from build123d import *

# Parameters (mm, degrees)
SKETCH1_W           = 38.1
SKETCH1_H           = 17.78
SKETCH1_R           = 1.778
BOSS_EXTRUDE2_DEPTH = 3.175
BOSS_EXTRUDE3_DEPTH = 38.1


with BuildPart() as part:
    # Sketch1 → Boss-Extrude2 (new body)
    with BuildSketch(Plane.XY):
        with Locations((19.05, -8.89)):
            Rectangle(SKETCH1_W, SKETCH1_H)
        with Locations((5.579618, -11.929615714)):
            Circle(SKETCH1_R, mode=Mode.SUBTRACT)
        with Locations((32.520382, -11.929615714)):
            Circle(SKETCH1_R, mode=Mode.SUBTRACT)
    extrude(amount=BOSS_EXTRUDE2_DEPTH)

    # Sketch4 → Boss-Extrude3 (add)
    with BuildSketch(Plane(origin=(38.1, 0, 0), x_dir=(0, 0, -1), z_dir=(1, 0, 0))):
        Polygon((-3.175, -6.35), (-15.875, 0), (-3.175, 0), align=None)
    extrude(amount=-BOSS_EXTRUDE3_DEPTH)


solid = part.part
Build history of the part. All positions in model axes, mm. Round coordinates to 2 decimals unless told otherwise and drop trailing zeros. Write each loop counter-clockwise with the first axis right and the second up, starting at its lowest first coordinate (ties: lowest second). Pieces come first, ordered by that corner, then holes. Notation, with made-up numbers: M 14.5,40.25 L 68.5,40.25 A34 ccw 68.5,77.25 Z; hole C 2,67 d8. An arc over 180 degrees is marked long. Answer as a JSON object with one key per item and string values. Group by question number.
(1) Cut at D-D (z = 10.75). Give the cut face in (x, y), and give its area (3 significant figures).
(2) Cut at C-C (y = -16.25). Give the cut face in (x, z) (3 decimals).
(3) Mould opens along X. For faces 1 (the flat face through (19, -12, 3.175)), 2 (the flat face through (38.1, -5, 4)), 3 (the cylindrical face through (4.27, -10.73, 1.57)) say: pulls with the +X half, pulls with the -X half, needs draft (parallel to the pull), parting line crosses it, or undercut.
(4) Drill centre lines: L1, parallel to X at y = -11, z = 1.5; L2, parallel to Z at x = 20, y = -16.75 (3 decimals); L3, parallel to Y at x = 4, z = 1.5. Where is each one in solid material? Low to high.
(5) Cut at A-A (z = 2.75). Give the cut face in (x, y).
(6) Cut at B-B (x = 21). Give the cut face in (y, z) (3 decimals).
(7) Flat gauge pins, fed straight in: pin 1 (2 mm diameter, centred on x = 15, z = 4.5, fed in from -Y); pin 2 (2 mm diameter, centred on x = 32.52, y = -11.93, fed in from +Z). Where does each tip first touch, or does it go through?
Responses:
{
 "1": {"outline": "M 0,-2.56 L 38.1,-2.56 L 38.1,0 L 0,0 Z", "area": "97.6 mm2"},
 "2": {"outline": "M 0,0 L 38.1,0 L 38.1,3.175 L 0,3.175 Z"},
 "3": {"face 1": "needs draft", "face 2": "pulls with the +X half", "face 3": "undercut"},
 "4": {"L1": "x = 0 to 4.06, 7.1 to 31, 34.04 to 38.1", "L2": "z = 0 to 3.175", "L3": "y = -17.78 to -12.75, -11.11 to 0"},
 "5": {"outline": "M 0,-17.78 L 38.1,-17.78 L 38.1,0 L 0,0 Z; hole C 5.58,-11.93 d3.56; hole C 32.52,-11.93 d3.56"},
 "6": {"outline": "M -17.78,0 L 0,0 L 0,15.875 L -6.35,3.175 L -17.78,3.175 Z"},
 "7": {"pin 1": "stops at y = -6.19", "pin 2": "passes through"}
}
